from build123d import *

# Parameters (mm, degrees)
SKETCH1_W                     = 104.775
SKETCH1_H                     = 106.3625
BOSS_EXTRUDE1_DEPTH           = 4
BOSS_EXTRUDE2_DEPTH           = 25
SKETCH3_R                     = 5
SKETCH3_R_2                   = 3.025
BOSS_EXTRUDE3_DEPTH           = 10
SKETCH4_R                     = 7
SKETCH4_R_2                   = 3.025
BOSS_EXTRUDE4_DEPTH           = 6.35
SKETCH6_W                     = 15.875
SKETCH6_H                     = 15.875
SKETCH6_W_2                   = 15.88
SKETCH6_H_2                   = 15.88
BOSS_EXTRUDE5_DEPTH           = 6
SKETCH8_W                     = 2.65
SKETCH8_H                     = 4
M5_CLEARANCE_HOLE2_AT_2_COUNT = 2
M5_CLEARANCE_HOLE2_AT_2_PITCH = 154.672014215
FILLET2_R                     = 3
CUT_EXTRUDE1_DEPTH            = 96.468237691


with BuildPart() as part:
    # Sketch1 → Boss-Extrude1 (new body)
    with BuildSketch(Plane.XY):
        Rectangle(SKETCH1_W, SKETCH1_H)
    extrude(amount=BOSS_EXTRUDE1_DEPTH)

    # Sketch2 → Boss-Extrude2 (add)
    with BuildSketch(Plane.XY):
        Polygon((-57.3875, -53.18125), (-57.3875, -58.18125), (-52.3875, -58.18125), (57.3875, -58.18125), (57.3875, 53.18125), (52.3875, 53.18125), (52.3875, -53.18125), (-52.3875, -53.18125), (-52.3875, 53.18125), (-57.3875, 53.18125), align=None)
    extrude(amount=BOSS_EXTRUDE2_DEPTH)

    # Sketch3 → Boss-Extrude3 (add)
    # profile 1 of 4: a face of its own
    with BuildSketch(Plane.XY.offset(4)):
        with Locations((43.708, 39.35095)):
            Circle(SKETCH3_R)
        with Locations((43.708, 39.35095)):
            Circle(SKETCH3_R_2, mode=Mode.SUBTRACT)
    # profile 2 of 4: a face of its own
    with BuildSketch(Plane.XY.offset(4)):
        with Locations((-41.382, 39.35095)):
            Circle(SKETCH3_R)
        with Locations((-41.382, 39.35095)):
            Circle(SKETCH3_R_2, mode=Mode.SUBTRACT)
    # profile 3 of 4: a face of its own
    with BuildSketch(Plane.XY.offset(4)):
        with Locations((-41.382, -47.00905)):
            Circle(SKETCH3_R)
        with Locations((-41.382, -47.00905)):
            Circle(SKETCH3_R_2, mode=Mode.SUBTRACT)
    # profile 4 of 4: a face of its own
    with BuildSketch(Plane.XY.offset(4)):
        with Locations((43.708, -47.00905)):
            Circle(SKETCH3_R)
        with Locations((43.708, -47.00905)):
            Circle(SKETCH3_R_2, mode=Mode.SUBTRACT)
    extrude(amount=BOSS_EXTRUDE3_DEPTH)

    # Sketch4 → Boss-Extrude4 (add)
    # profile 1 of 4: a face of its own
    with BuildSketch(Plane.XY.offset(4)):
        with Locations((43.708, 39.35095)):
            Circle(SKETCH4_R)
        with Locations((43.708, 39.35095)):
            Circle(SKETCH4_R_2, mode=Mode.SUBTRACT)
    # profile 2 of 4: a face of its own
    with BuildSketch(Plane.XY.offset(4)):
        with Locations((-41.382, 39.35095)):
            Circle(SKETCH4_R)
        with Locations((-41.382, 39.35095)):
            Circle(SKETCH4_R_2, mode=Mode.SUBTRACT)
    # profile 3 of 4: a face of its own
    with BuildSketch(Plane.XY.offset(4)):
        with Locations((-41.382, -47.00905)):
            Circle(SKETCH4_R)
        with Locations((-41.382, -47.00905)):
            Circle(SKETCH4_R_2, mode=Mode.SUBTRACT)
    # profile 4 of 4: a face of its own
    with BuildSketch(Plane.XY.offset(4)):
        with Locations((43.708, -47.00905)):
            Circle(SKETCH4_R)
        with Locations((43.708, -47.00905)):
            Circle(SKETCH4_R_2, mode=Mode.SUBTRACT)
    extrude(amount=BOSS_EXTRUDE4_DEPTH)

    # Sketch6 → Boss-Extrude5 (add)
    with BuildSketch(Plane.XY):
        with Locations((65.325, 32.54375)):
            Rectangle(SKETCH6_W, SKETCH6_H)
        with Locations((-65.3275, -50.24125)):
            Rectangle(SKETCH6_W_2, SKETCH6_H_2)
    extrude(amount=BOSS_EXTRUDE5_DEPTH)

    # Sketch8 → M5 Clearance Hole2 (revolve, cut)
    with BuildSketch(Plane(origin=(65.325, 32.54375, 4), x_dir=(0, -1, 0), z_dir=(1, 0, 0))):
        with Locations((1.325, 2)):
            Rectangle(SKETCH8_W, SKETCH8_H)
    m5_clearance_hole2 = revolve(axis=Axis((65.325, 32.54375, 10.35), (0, 0, -1)), mode=Mode.SUBTRACT)

    # M5 Clearance Hole2 at 2: M5 Clearance Hole2 ×2
    with Locations(*[Vector(-0.8447067859256896, -0.5352293394528098, 0) * (i * M5_CLEARANCE_HOLE2_AT_2_PITCH) for i in range(1, M5_CLEARANCE_HOLE2_AT_2_COUNT)]):
        add(m5_clearance_hole2, mode=Mode.SUBTRACT)

    # Fillet2
    fillet2_edges = [part.edges().sort_by_distance(p)[0] for p in [
        (-73.2675, -42.30125, 3),
        (-73.2675, -58.18125, 3),
        (73.2625, 24.60625, 3),
        (73.2625, 40.48125, 3),
        (57.3875, 40.48125, 3),
        (57.3875, 24.60625, 3),
    ]]
    fillet(fillet2_edges, radius=FILLET2_R)

    # Sketch11 → Cut-Extrude1 (cut, through all)
    with BuildSketch(Plane.XY.offset(6)):
        with BuildLine():
            Line((-67.9775, -42.30125), (-67.9775, -50.24125))
            ThreePointArc((-67.9775, -50.24125), (-65.3275, -47.59125), (-62.6775, -50.24125))
            Line((-62.6775, -50.24125), (-62.6775, -42.30125))
            Line((-62.6775, -42.30125), (-67.9775, -42.30125))
        make_face()
        with BuildLine():
            Line((62.675, 40.48125), (62.675, 32.54375))
            ThreePointArc((62.675, 32.54375), (65.325, 35.19375), (67.975, 32.54375))
            Line((67.975, 32.54375), (67.975, 40.48125))
            Line((67.975, 40.48125), (62.675, 40.48125))
        make_face()
    extrude(amount=-CUT_EXTRUDE1_DEPTH, mode=Mode.SUBTRACT)


solid = part.part
Verification items for the finished model (mm, model axes). A direction names the side the tool comes from. Round coordinates to 2 decimals unless told otherwise and drop trailing zeros. Order: outer loops, then holes, each group sorted by start corner. A loop starts at its lowest first (then second) coordinate and runs counter-clockwise, first axis right, second up.
1. Section check C-C on x = -10.5. Record the cut outline in (y, z), then the cut area to 3 significant figures.
Final values:
outline: (-58.18, 0) - (53.18, 0) - (53.18, 4) - (-53.18, 4) - (-53.18, 25) - (-58.18, 25) - close
area: 550 mm2
2. Release check for a two-part mould opening along X. For faces 1 (the cylindrical face through (-72.41, -57.28, 3.04)), 2 (the cylindrical face through (-39.075, -51.445, 12.149)), 3 (the flat face through (-60, -42.301, 3)) record: +X half, -X half, draft (parallel to the pull), parting line (faces both ways), or undercut.
Final values:
face 1: -X half
face 2: undercut
face 3: draft
3. Access from +Z, -Z, +X, -X, +Y, -Y to the whole of each face (thin tool, end or side, straight path). Record for faces 4 (the cylindrical face through (43.06, 44.31, 12.15)), 5 (the flat face through (-65, -50, 6)), 6 (the flat face through (46, 37, 14)), 7 (the cylindrical face through (65.383, 29.894, 1.972)), 8 (the flat face through (-7, -58.181, 12)).
Final values:
face 4: +Z
face 5: +Z, -X, +Y, -Y
face 6: +Z, +Y
face 7: -Z, +Y
face 8: +Z, -Z, +X, -X, -Y
4. Section check B-B on z = 16.5. Record the cut outline in (x, y).
Final values:
outline: (-57.39, -58.18) - (57.39, -58.18) - (57.39, 53.18) - (52.39, 53.18) - (52.39, -53.18) - (-52.39, -53.18) - (-52.39, 53.18) - (-57.39, 53.18) - close
5. Thickness scan on L1, parallel to X at y = -26, z = 18.75; L2, parallel to Y at x = -43.5, z = 12; L3, parallel to Z at x = 30.5, y = -17.5. Record the ranges inside material, lowest first.
Final values:
L1: x = -57.39 to -52.39, 52.39 to 57.39
L2: y = -58.18 to -53.18, -51.54 to -49.17, -44.85 to -42.48, 34.82 to 37.19, 41.51 to 43.88
L3: z = 0 to 4
6. Section check A-A on y = -21. Record the cut outline in (x, z), then the cut area to 3 significant figures.
Final values:
outline: (-57.39, 0) - (57.39, 0) - (57.39, 25) - (52.39, 25) - (52.39, 4) - (-52.39, 4) - (-52.39, 25) - (-57.39, 25) - close
area: 669 mm2
7. Go/stop test with flat-tipped pins: P1, Ø5, axis at x = 43.71, y = -47.01, coming from the +Z side; P2, Ø1, axis at y = 9.5, z = 9, coming from the -X side; P3, Ø2, axis at x = -42.5, z = 6, coming from the +Y side. Record where each tip stops, or that it passes through.
Final values:
P1: stops at z = 4
P2: stops at x = -57.39
P3: stops at y = 46.35
